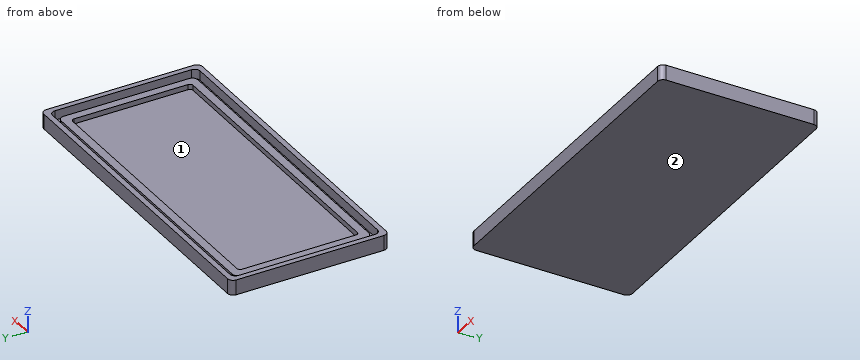
Solid Edge part; units mm, degrees
sketch "Sketch1" plane through (0, 0, 0) normal (0, 0, 1) x (1, 0, 0)
  line L0 (-60, 29) -> (60, 29)
  line L1 (60, 29) -> (60, -29)
  line L2 (60, -29) -> (-60, -29)
  line L3 (-60, -29) -> (-60, 29)
  dimension "D1" = 60
  dimension "D2" = 60
extrude "Protrusion1" add sketch "Sketch1" along normal blind 5.5
fillet "Redondo_1" radius 2 4 edges at (60, 29, 2.75) (60, -29, 2.75) (-60, 29, 2.75) (-60, -29, 2.75)
sketch "Sketch2" plane through (0, 0, 5.5) normal (0, 0, 1) x (1, 0, 0)
  line L0 (-56, 27) -> (56, 27)
  arc A0 (56, 27) -> (58, 25) centre (56, 25) cw
  line L1 (58, 25) -> (58, -25)
  arc A1 (56, -27) -> (58, -25) centre (56, -25) ccw
  line L2 (56, -27) -> (-56, -27)
  arc A2 (-56, -27) -> (-58, -25) centre (-56, -25) cw
  line L3 (-58, -25) -> (-58, 25)
  arc A3 (-56, 27) -> (-58, 25) centre (-56, 25) ccw
extrude "Recorte_Extrudado_1" cut sketch "Sketch2" against normal blind 3.5
sketch "Sketch3" plane through (0, 0, 2) normal (0, 0, 1) x (1, 0, 0)
  line L0 (-54, 25) -> (54, 25)
  arc A0 (54, 25) -> (56, 23) centre (54, 23) cw
  line L1 (56, 23) -> (56, -23)
  arc A1 (56, -23) -> (54, -25) centre (54, -23) cw
  line L2 (54, -25) -> (-54, -25)
  arc A2 (-56, -23) -> (-54, -25) centre (-54, -23) ccw
  line L3 (-56, -23) -> (-56, 23)
  arc A3 (-56, 23) -> (-54, 25) centre (-54, 23) cw
  line L4 (-51.8587, 22) -> (51.8587, 22)
  arc A4 (53, 20.8587) -> (51.8587, 22) centre (51.8587, 20.8587) ccw
  line L5 (53, 20.8587) -> (53, -20.8587)
  arc A5 (51.8587, -22) -> (53, -20.8587) centre (51.8587, -20.8587) ccw
  line L6 (51.8587, -22) -> (-51.8587, -22)
  arc A6 (-51.8587, -22) -> (-53, -20.8587) centre (-51.8587, -20.8587) cw
  line L7 (-53, -20.8587) -> (-53, 20.8587)
  arc A7 (-53, 20.8587) -> (-51.8587, 22) centre (-51.8587, 20.8587) cw
extrude "Protrusion2" add sketch "Sketch3" along normal blind 1.9
The listing builds one solid part. Answer for the finished solid, in the listing's coordinates (mm). Face numbers are marked on the shaded views. Give positions to 0.01 mm unless a question says otherwise; leave off trailing zeros. Write each loop counter-clockwise with the first axis right and the second up, starting at its lowest first coordinate (ties: lowest second). Pieces come first, ordered by that corner, then holes. Notation, with made-up numbers: (48, -23) -> (88, -23) arc R14 cw to (88, 3) -> close; hole circle Ø2 at (20.5, 78). An arc over 180 degrees is marked (long way). Use a Markdown table: item, result.
(1) Section A-A, the plane x = -32 is taken. Determine the outline of the cut face in (y, z), then the cut area to 3 significant figures.
Return value:
| item | result |
|---|---|
| outline | (-29, 0) -> (29, 0) -> (29, 5.5) -> (27, 5.5) -> (27, 2) -> (25, 2) -> (25, 3.9) -> (22, 3.9) -> (22, 2) -> (-22, 2) -> (-22, 3.9) -> (-25, 3.9) -> (-25, 2) -> (-27, 2) -> (-27, 5.5) -> (-29, 5.5) -> close |
| area | 141 mm2 |
(2) Find the intervals of material crossed by probe 1 along Y at (x, z) = (-17, 3.35); probe 2 along X at (y, z) = (16, 2.45); probe 3 along Y at (x, z) = (-4, 4.7), in increasing order. Write a range as from..to.
Return value:
| item | result |
|---|---|
| probe 1 | -29..-27, -25..-22, 22..25, 27..29 |
| probe 2 | -60..-58, -56..-53, 53..56, 58..60 |
| probe 3 | -29..-27, 27..29 |
(3) Determine the mould class of the marked faces 1 and 2 for opening direction Y: released by +Y, released by -Y, zero draft, split by the parting line, or undercut.
Return value:
| item | result |
|---|---|
| face 1 | undercut |
| face 2 | zero draft |
(4) Section B-B, the plane y = -10.5 is taken. Determine the outline of the cut face in (x, z).
Return value:
| item | result |
|---|---|
| outline | (-60, 0) -> (60, 0) -> (60, 5.5) -> (58, 5.5) -> (58, 2) -> (56, 2) -> (56, 3.9) -> (53, 3.9) -> (53, 2) -> (-53, 2) -> (-53, 3.9) -> (-56, 3.9) -> (-56, 2) -> (-58, 2) -> (-58, 5.5) -> (-60, 5.5) -> close |
(5) A flat-ended cylindrical pin translates along its axis: P1, Ø16, axis at x = 5, y = 10.5, coming from the +Z side. Find the tip coordinate at first contact, or state that the pin passes through.
Return value:
| item | result |
|---|---|
| P1 | z = 2 |
